```python
from build123d import *

# Parameters (mm, degrees)
F0_R     = 10.5
F1_DEPTH = 4
F2_R     = 8
F3_DEPTH = 39


# Not quite as in the source:
# - a feature names something its author has since deleted; it is built from what else it names


with BuildPart() as f1:
    # F0 (on Top) → F1 (new body)
    with BuildSketch(Plane.XY):
        Circle(F0_R)
    extrude(amount=F1_DEPTH)

    # F2 (on Top) → F3 (join)
    with BuildSketch(Plane.XY):
        Circle(F2_R)
    extrude(amount=F3_DEPTH)

    # F4 (on Right) → F5 (revolve)
    with BuildSketch(Plane.YZ):
        with BuildLine():
            ThreePointArc((5, 39), (3.5355339059, 42.5355339059), (0, 44))
            Line((0, 44), (0, 39))
            Line((0, 39), (5, 39))
        make_face()
    revolve(axis=Axis((0, 0, 41.5), (0, 0, -1)))


solid = f1.part
```
The listing builds one solid part. Answer for the finished solid, in the listing's coordinates (mm). A direction names the side the tool comes from. Coordinates: 2 decimals unless noted, no trailing zeros. Write each loop counter-clockwise with the first axis right and the second up, starting at its lowest first coordinate (ties: lowest second). Pieces come first, ordered by that corner, then holes. Notation, with made-up numbers: (85, 49.5) - (96, 49.5) arc R25 ccw to (96, 77.5) - close; hole circle Ø11 at (68.5, 53). An arc over 180 degrees is marked (long way). Return JSON: item names as keys, results as strings. Group by question number.
Q1. Flat-ended cylindrical pins translate along their axes: pin 1 Ø6 at (y, z) = (-6, 20) entering from +X; pin 2 Ø1.5 at (x, z) = (-3, 18) entering from +Y; pin 3 Ø5 at (x, y) = (-4, 1) entering from +Z. Find the tip coordinate at first contact, or state that the pin passes through.
Q2. The part is cut by section C-C on z = 3.5. Write down the section's boundary in (x, y).
Q3. Find the intervals of material crossed by line 1 along Z through (x, y) = (-7, 7.5); line 2 along Z through (x, y) = (3, 5); line 3 along Y through (x, z) = (0.25, 29), in increasing order. Write a range as [from, to].
Q4. The part is cut by section D-D on x = 6. Write down the section's boundary in (y, z), and give its area (3 significant figures).
Q5. The part is cut by section A-A on y = 0. Write down the section's boundary in (x, z), and give its area (3 significant figures).
Q6. Which of the six approach directions +Z, -Z, +X, -X, +Y, -Y give full straight-line access (tool end or side, diameter ignored) to faces 1 (the flat face through (-2, -8, 4)), 2 (the cylindrical face through (10, 3.2, 2))?
Evaluation:
{
 "1": {"pin 1": "stops at x = 7.42", "pin 2": "stops at y = 7.68", "pin 3": "stops at z = 43.73"},
 "2": {"outline": "circle Ø21 at (0, 0)"},
 "3": {"line 1": "z = [0, 4]", "line 2": "z = [0, 39]", "line 3": "y = [-8, 8]"},
 "4": {"outline": "(-8.62, 0) - (8.62, 0) - (8.62, 4) - (5.29, 4) - (5.29, 39) - (-5.29, 39) - (-5.29, 4) - (-8.62, 4) - close", "area": "439 mm2"},
 "5": {"outline": "(-10.5, 0) - (10.5, 0) - (10.5, 4) - (8, 4) - (8, 39) - (5, 39) arc R5 ccw to (-5, 39) - (-8, 39) - (-8, 4) - (-10.5, 4) - close", "area": "683 mm2"},
 "6": {"face 1": "+Z", "face 2": "+Z, -Z"}
}
